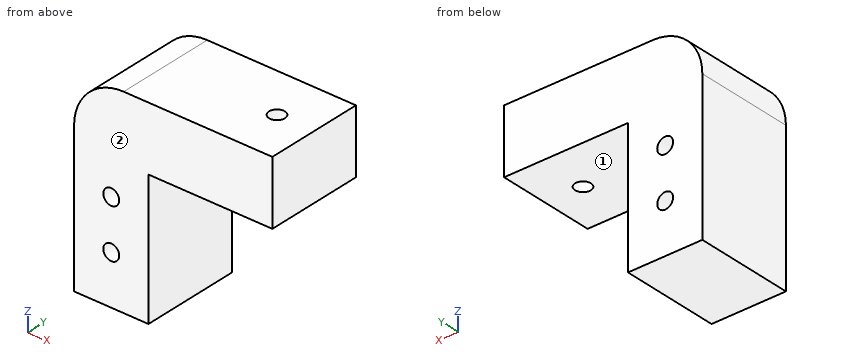
from build123d import *

# Parameters (mm, degrees)
SKETCH_1_W          = 40
SKETCH_1_H          = 40
SKETCH_1_R          = 1.6
EXTRUDE_1_DEPTH     = 20
SKETCH_2_R          = 1.6
CUT_EXTRUDE_1_DEPTH = 61
SKETCH_3_W          = 25
SKETCH_3_H          = 20
CUT_EXTRUDE_2_DEPTH = 27
FILLET_1_R          = 10


with BuildPart() as part:
    # 草图1 → 凸台-拉伸1 (new body)
    with BuildSketch(Plane(origin=(0, 0, 0), x_dir=(1, 0, 0), z_dir=(0, 1, 0))):
        with Locations((20, 20)):
            Rectangle(SKETCH_1_W, SKETCH_1_H)
        with Locations(Location((7.5, 30, 0), (0, 0, 270))):
            Circle(SKETCH_1_R, mode=Mode.SUBTRACT)
        with Locations(Location((7.5, 20, 0), (0, 0, 270))):
            Circle(SKETCH_1_R, mode=Mode.SUBTRACT)
    extrude(amount=EXTRUDE_1_DEPTH)

    # 草图2 → 切除-拉伸1 (cut, through all)
    with BuildSketch(Plane(origin=(0, 0, -40), x_dir=(-1, 0, 0), z_dir=(0, 0, -1))):
        with Locations((-32.5, 10)):
            Circle(SKETCH_2_R)
    extrude(amount=-CUT_EXTRUDE_1_DEPTH, mode=Mode.SUBTRACT)

    # 草图3 → 切除-拉伸2 (cut)
    with BuildSketch(Plane(origin=(0, 0, -40), x_dir=(-1, 0, 0), z_dir=(0, 0, -1))):
        with Locations((-27.5, 10)):
            Rectangle(SKETCH_3_W, SKETCH_3_H)
    extrude(amount=-CUT_EXTRUDE_2_DEPTH, mode=Mode.SUBTRACT)

    # 圆角1
    fillet_1_edges = [part.edges().sort_by_distance(p)[0] for p in [
        (0, 10, 0),
    ]]
    fillet(fillet_1_edges, radius=FILLET_1_R)


solid = part.part
Could you check a few things on this model? Use its own coordinates, in mm. Face numbers are marked on the shaded views. A direction names the side the tool comes from. Give positions to 0.01 mm unless a question says otherwise; leave off trailing zeros. Loops run counter-clockwise (first coordinate to the right, second up) from the corner with the lowest first, then second, coordinate; pieces in that order, holes last. Notation, with made-up numbers: (86, 20) -> (97, 20) arc R23 ccw to (97, 39) -> close; hole circle Ø8 at (75.5, -16.75). An arc over 180 degrees is marked (long way). Answer as CSV lines item,"result". Start each with the question number.
(1) I'm going to push flat-ended pins straight in: pin 1 Ø6 at (x, y) = (25, 14.5) entering from -Z; pin 2 Ø10 at (y, z) = (9, -32.5) entering from +X; pin 3 Ø3.5 at (x, z) = (7.5, -20) entering from +Y; pin 4 Ø2.5 at (x, z) = (7.5, -30) entering from -Y. Where does each tip first touch, or does it pass through?
(2) If we section it at B-B on x = 32.5: Write out the boundary of the cut face in (y, z), then the cut area to 3 significant figures.
(3) I need wall thicknesses on probe 1 along X at (y, z) = (4.75, -20); probe 2 along X at (y, z) = (11.25, -18); probe 3 along Z at (x, y) = (32, 18.25). Which ranges of each line are inside material? Lowest first, please.
(4) If we section it at C-C on z = -20: Write out the boundary of the cut face in (x, y), then the cut area to 3 significant figures.
(5) If we section it at D-D on y = 7: Write out the boundary of the cut face in (x, z), then the cut area to 3 significant figures.
(6) If we section it at A-A on y = 10: Write out the boundary of the cut face in (x, z), then the cut area to 3 significant figures.
(7) Which directions (+Z, -Z, +X, -X, +Y, -Y) give clear straight access to the entire face, cutting with the end or side of a thin tool? Please do the marked faces 1 and 2.
Computed:
1,pin 1,"stops at z = -13"
1,pin 2,"stops at x = 15"
1,pin 3,"stops at y = 20"
1,pin 4,"passes through"
2,outline,"(0, -13) -> (8.4, -13) -> (8.4, 0) -> (0, 0) -> close; (11.6, -13) -> (20, -13) -> (20, 0) -> (11.6, 0) -> close"
2,area,"218 mm2"
3,probe 1,"x = 0 to 5.9, 9.1 to 15"
3,probe 2,"x = 0 to 15"
3,probe 3,"z = -13 to 0"
4,outline,"(0, 0) -> (5.9, 0) -> (5.9, 20) -> (0, 20) -> close; (9.1, 0) -> (15, 0) -> (15, 20) -> (9.1, 20) -> close"
4,area,"236 mm2"
5,outline,"(0, -40) -> (15, -40) -> (15, -13) -> (40, -13) -> (40, 0) -> (10, 0) arc R10 ccw to (0, -10) -> close; hole circle Ø3.2 at (7.5, -30); hole circle Ø3.2 at (7.5, -20)"
5,area,"887 mm2"
6,outline,"(0, -40) -> (15, -40) -> (15, -13) -> (30.9, -13) -> (30.9, 0) -> (10, 0) arc R10 ccw to (0, -10) -> close; (34.1, -13) -> (40, -13) -> (40, 0) -> (34.1, 0) -> close; hole circle Ø3.2 at (7.5, -30); hole circle Ø3.2 at (7.5, -20)"
6,area,"846 mm2"
7,face 1,"-Z, +X, +Y, -Y"
7,face 2,"+Z, -Z, +X, -X, -Y"
